Part model, mm, in its own coordinate system. A direction names the side the tool comes from. Round coordinates to 2 decimals unless told otherwise and drop trailing zeros. Loops run counter-clockwise (first coordinate to the right, second up) from the corner with the lowest first, then second, coordinate; pieces in that order, holes last.
1) Drop flat-ended pins along their axis: P1, Ø7.5, axis at x = -19, z = 9, coming from the +Y side; P2, Ø2.5, axis at y = 1.5, z = 13, coming from the -X side; P3, Ø3.5, axis at y = -7.5, z = 6.5, coming from the -X side. Give the stop position or say it passes through.
2) Band-saw the part on B-B, the plane x = 31. Write the cut outline in (y, z), then the cut area to 3 significant figures.
3) Band-saw the part on C-C, the plane y = -5.5. Write the cut outline in (x, z), then the cut area to 3 significant figures.
4) 3-axis set-ups, long thin cutter, end or side, ignore diameter. For faces 1 (the flat face through (37, 0, 12)), 2 (the flat face through (-47, -11.84, 12)), 3 (the flat face through (-1, -17.177, 12)): which of +Z, -Z, +X, -X, +Y, -Y reach the whole face in a straight line?
5) Band-saw the part on A-A, the plane z = 10.25. Write the cut outline in (x, y), then the cut area to 3 significant figures.
6) Probe line 1 (X direction, y = -11.25, z = 12); line 2 (Y direction, x = 38.5, z = 16.25); line 3 (Y direction, x = -43.5, z = 20). List the from-to ranges inside material, lowest first.
from build123d import *

# Parameters (mm, degrees)
F0_W     = 9.444609
F0_H     = 13.117496
F1_DEPTH = 25


with BuildPart() as f1:
    # F0 (on Top) → F1 (new body)
    with BuildSketch(Plane.XY):
        with Locations((48.95623, -10.61799)):
            Rectangle(F0_W, F0_H)
        Polygon((19.53455, 0), (44.233926, -17.176738), (44.233926, -4.059242), (53.678535, -4.059242), (49.502895, 0), align=None)
        Polygon((-53.678535, -17.176738), (44.233926, -17.176738), (19.53455, 0), (16.513675, 0), (11.002047, 0), (-24.868423, 0), (-41.03421, 0), (-41.03421, -11.840364), (-53.678535, -11.840364), align=None)
        Polygon((49.502895, 0), (53.678535, -4.059242), (53.678535, 0), align=None)
        Polygon((16.513675, 0), (19.53455, 0), (16.513675, 2.100813), align=None)
    extrude(amount=F1_DEPTH)


solid = f1.part
Reported:
1. P1: stops at y = 0
1. P2: stops at x = 16.51
1. P3: stops at x = -41.03
2. outline: (-17.18, 0) - (0, 0) - (0, 25) - (-17.18, 25) - close
2. area: 429 mm2
3. outline: (-41.03, 0) - (53.68, 0) - (53.68, 25) - (-41.03, 25) - close
3. area: 2,370 mm2
4. face 1: +Z, -Z, +X, +Y
4. face 2: +Z, -Z, -X, +Y
4. face 3: +Z, -Z, +X, -X, -Y
5. outline: (-53.68, -17.18) - (53.68, -17.18) - (53.68, 0) - (19.53, 0) - (16.51, 2.1) - (16.51, 0) - (-41.03, 0) - (-41.03, -11.84) - (-53.68, -11.84) - close
5. area: 1,700 mm2
6. line 1: x = -41.03 to 53.68
6. line 2: y = -17.18 to 0
6. line 3: y = -17.18 to -11.84
